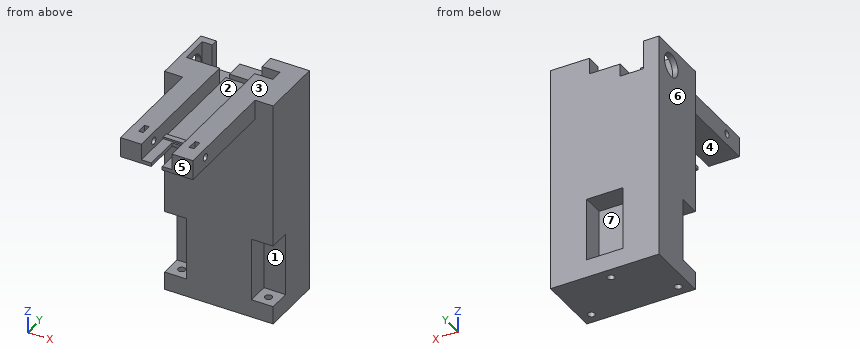
from build123d import *

# Parameters (mm, degrees)
F0_W      = 60
F0_H      = 35
F0_R      = 2
F1_DEPTH  = 10
F3_DEPTH  = 35
F4_W      = 60
F4_H      = 35
F5_DEPTH  = 70
F7_DEPTH  = 2
F9_DEPTH  = 1
F11_DEPTH = 8
F12_R     = 2
F13_DEPTH = 45
F14_W     = 2.6
F14_H     = 5.7
F15_DEPTH = 8.7
F18_DEPTH = 16
F19_R     = 6.5
F20_DEPTH = 5
F22_W     = 3
F22_H     = 7
F23_DEPTH = 12
F24_DEPTH = 5


with BuildPart() as f1:
    # F0 (on Top) → F1 (new body)
    with BuildSketch(Plane.XY):
        Rectangle(F0_W, F0_H)
        with Locations((-24, -11.5)):
            Circle(F0_R, mode=Mode.SUBTRACT)
        with Locations((24, -11.5)):
            Circle(F0_R, mode=Mode.SUBTRACT)
        with Locations((0, 11.5)):
            Circle(F0_R, mode=Mode.SUBTRACT)
    extrude(amount=F1_DEPTH)

    # F2 (on face) → F3 (join)
    with BuildSketch(Plane.XY.offset(10)):
        Polygon((-10, 17.5), (-30, 17.5), (-30, -5.5), (-18, -5.5), (-18, -17.5), (18, -17.5), (18, -5.5), (30, -5.5), (30, 17.5), (10, 17.5), (10, 5.5), (-10, 5.5), align=None)
    extrude(amount=F3_DEPTH)

    # F4 (on face) → F5 (join)
    with BuildSketch(Plane.XY.offset(45)):
        Rectangle(F4_W, F4_H)
    extrude(amount=F5_DEPTH)

    # F6 (on face) → F7 (join)
    with BuildSketch(Plane.XY.offset(115)):
        Polygon((30, 17.5), (-30, 17.5), (-30, -17.5), (-20, -17.5), (-20, -77.5), (-3, -77.5), (-3, -57.5), (3, -57.5), (3, -77.5), (20, -77.5), (20, -17.5), (30, -17.5), align=None)
    extrude(amount=F7_DEPTH)

    # F8 (on face) → F9 (join)
    with BuildSketch(Plane.XY.offset(117)):
        Polygon((-30, 17.5), (-30, -17.5), (-20, -17.5), (-20, -77.5), (-8.5, -77.5), (-8.5, -56.5), (8.5, -56.5), (8.5, -77.5), (20, -77.5), (20, -17.5), (30, -17.5), (30, 17.5), (8.5, 17.5), (8.5, -53.5), (-8.5, -53.5), (-8.5, 17.5), align=None)
    extrude(amount=F9_DEPTH)

    # F10 (on face) → F11 (join)
    with BuildSketch(Plane.XY.offset(118)):
        Polygon((-20, -77.5), (-8.5, -77.5), (-8.5, 17.5), (-30, 17.5), (-30, -17.5), (-20, -17.5), align=None)
        Polygon((8.5, -77.5), (20, -77.5), (20, -17.5), (30, -17.5), (30, 17.5), (8.5, 17.5), align=None)
    extrude(amount=F11_DEPTH)

    # F12 (on face) → F13 (cut)
    with BuildSketch(Plane.YZ.offset(20)):
        with Locations((-65.5104211917, 121)):
            Circle(F12_R)
    extrude(amount=-F13_DEPTH, mode=Mode.SUBTRACT)

    # F14 (on face) → F15 (cut)
    with BuildSketch(Plane.XY.offset(126)):
        with Locations((14, -65.5)):
            Rectangle(F14_W, F14_H)
        with Locations((-14, -65.5)):
            Rectangle(F14_W, F14_H)
    extrude(amount=-F15_DEPTH, mode=Mode.SUBTRACT)

    # F17 (on offset) → F18 (cut)
    with BuildSketch(Plane.XY.offset(110)):
        Polygon((-21.5, 13.5), (-27, 13.5), (-27, -2), (-8.5, -2), (-8.5, 4), (8.5, 4), (8.5, 2.25), (15.5, 2.25), (15.5, 9.25), (8.5, 9.25), (8.5, 7.5), (-8.5, 7.5), (-8.5, 13.5), (-8.5, 17.5), (-21.5, 17.5), align=None)
    extrude(amount=F18_DEPTH, mode=Mode.SUBTRACT)

    # F19 (on face) → F20 (cut)
    with BuildSketch(Plane.YZ.offset(-27)):
        with Locations((5.75, 116)):
            Circle(F19_R)
    extrude(amount=-F20_DEPTH, mode=Mode.SUBTRACT)

    # F22 (on offset) → F23 (cut)
    with BuildSketch(Plane.XY.offset(114)):
        with Locations((17, 5.75)):
            Rectangle(F22_W, F22_H)
    extrude(amount=F23_DEPTH, mode=Mode.SUBTRACT)

    # F22 (on offset) → F24 (join)
    with BuildSketch(Plane.XY.offset(114)):
        with Locations((17, 5.75)):
            Rectangle(F22_W, F22_H)
    extrude(amount=F24_DEPTH)


solid = f1.part
The listing builds one solid part. Answer for the finished solid, in the listing's coordinates (mm). Face numbers are marked on the shaded views. A direction names the side the tool comes from. Coordinates: 2 decimals unless noted, no trailing zeros. Write each loop counter-clockwise with the first axis right and the second up, starting at its lowest first coordinate (ties: lowest second). Pieces come first, ordered by that corner, then holes. Notation, with made-up numbers: (-19.75, -35) - (4.25, -35) arc R25 ccw to (4.25, -16) - close; hole circle Ø9 at (49.25, -23). An arc over 180 degrees is marked (long way). Return JSON: item names as keys, results as strings.
1. The part is cut by section B-B on x = 0. Determine the outline of the cut face in (y, z).
Final values:
{"outline": "(-57.5, 115) - (-17.5, 115) - (-17.5, 0) - (9.5, 0) - (9.5, 10) - (5.5, 10) - (5.5, 45) - (17.5, 45) - (17.5, 117) - (7.5, 117) - (7.5, 110) - (4, 110) - (4, 117) - (-53.5, 117) - (-53.5, 118) - (-56.5, 118) - (-56.5, 117) - (-57.5, 117) - close; (13.5, 0) - (17.5, 0) - (17.5, 10) - (13.5, 10) - close"}
2. The part is cut by section A-A on y = -11.5. Determine the outline of the cut face in (x, z).
Final values:
{"outline": "(-30, 0) - (-26, 0) - (-26, 10) - (-30, 10) - close; (-30, 45) - (-18, 45) - (-18, 10) - (-22, 10) - (-22, 0) - (22, 0) - (22, 10) - (18, 10) - (18, 45) - (30, 45) - (30, 126) - (8.5, 126) - (8.5, 117) - (-8.5, 117) - (-8.5, 126) - (-30, 126) - close; (26, 0) - (30, 0) - (30, 10) - (26, 10) - close"}
3. Consider line 1 along Y through (x, z) = (0, 3); line 2 along Z through (x, y) = (-29.35, 5.75); line 3 along Y through (x, z) = (13, 117). Determine where each line is inside the solid, lowest interval first.
Final values:
{"line 1": "-17.5 to 9.5, 13.5 to 17.5", "line 2": "0 to 109.5, 122.5 to 126", "line 3": "-77.5 to 2.25, 9.25 to 17.5"}
4. Each of these flat-tipped pins is pushed along its axis until it touches: pin 1 Ø0.5 at (x, z) = (-3.5, 117.5) entering from -Y; pin 2 Ø11.5 at (y, z) = (5.75, 116) entering from -X; pin 3 Ø5 at (y, z) = (-65.51, 121) entering from -X. Where does it stop, or does it pass through?
Final values:
{"pin 1": "y = -56.5", "pin 2": "x = -8.5", "pin 3": "x = -20"}
5. The part is cut by section D-D on x = -24. Determine the outline of the cut face in (y, z), then the cut area to 3 significant figures.
Final values:
{"outline": "(-17.5, 0) - (-13.5, 0) - (-13.5, 10) - (-17.5, 10) - close; (-17.5, 45) - (-5.5, 45) - (-5.5, 10) - (-9.5, 10) - (-9.5, 0) - (17.5, 0) - (17.5, 126) - (13.5, 126) - (13.5, 110) - (-2, 110) - (-2, 126) - (-17.5, 126) - close", "area": "3,700 mm^2"}
6. The part is cut by section C-C on z = 13. Determine the outline of the cut face in (x, y).
Final values:
{"outline": "(-30, -5.5) - (-18, -5.5) - (-18, -17.5) - (18, -17.5) - (18, -5.5) - (30, -5.5) - (30, 17.5) - (10, 17.5) - (10, 5.5) - (-10, 5.5) - (-10, 17.5) - (-30, 17.5) - close"}
7. For a pull along X with two mould halves and no side action, classify the marked faces 5, 6 and 7 as +X half, -X half, draft (parallel to the pull), parting line (faces both ways), or undercut.
Final values:
{"face 5": "draft", "face 6": "-X half", "face 7": "undercut"}
8. Which of the six approach directions +Z, -Z, +X, -X, +Y, -Y give full straight-line access (tool end or side, diameter ignored) to the marked faces 1, 2, 3 and 4?
Final values:
{"face 1": "+X, -Y", "face 2": "+Z, +Y", "face 3": "+Z, +X, -X, +Y, -Y", "face 4": "-Z, +X, -X, -Y"}
